```python
from build123d import *

# Parameters (mm, degrees)
F0_R     = 3
F1_DEPTH = 10
F2_R     = 2.44
F3_DEPTH = 6
F4_R     = 2.7
F5_DEPTH = 5


with BuildPart() as f1:
    # F0 (on Top) → F1 (new body)
    with BuildSketch(Plane.XY):
        with Locations((-39.492015, 19.486886)):
            Circle(F0_R)
    extrude(amount=F1_DEPTH)

    # F2 (on face) → F3 (join)
    with BuildSketch(Plane.XY.offset(10)):
        with Locations((-39.492015, 19.486886)):
            Circle(F2_R)
    extrude(amount=F3_DEPTH)

    # F4 (on face) → F5 (cut)
    with BuildSketch(Plane(origin=(0, 0, 0), x_dir=(1, 0, 0), z_dir=(0, 0, -1))):
        with Locations((-39.492015, -19.486886)):
            Circle(F4_R)
    extrude(amount=-F5_DEPTH, mode=Mode.SUBTRACT)


solid = f1.part
```
Input: part model. Units: mm. Frame: model coordinates. Give positions to 0.01 mm unless a question says otherwise; leave off trailing zeros. Order: outer loops, then holes, each group sorted by start corner. A loop starts at its lowest first (then second) coordinate and runs counter-clockwise, first axis right, second up. Notation, with made-up numbers: M -23.5,8 L 33.5,8 A16 ccw 33.5,23 Z; hole C 49,-21.5 d10. An arc over 180 degrees is marked long. One line per question, with ' | ' between items. Start each with the question number.
1. Section query B-B (y = 21.6). Return the cut outline in (x, z).
2. Section query C-C (z = 4). Return the cut outline in (x, y).
3. Section query D-D (z = 13). Return the cut outline in (x, y), and give its area (3 significant figures).
4. First-contact query: pin 1 Ø3 at (x, z) = (-41, 13) entering from -Y; pin 2 Ø1 at (x, z) = (-40, 1.5) entering from -Y. Flat tips, straight axial feed; report the tip coordinate or a pass-through.
5. Section query A-A (x = -39.05). Return the cut outline in (y, z).
6. Material intervals for probe 1 along X at (y, z) = (19.6, 1.5); probe 2 along Z at (x, y) = (-40.8, 21.75); probe 3 along X at (y, z) = (18.15, 4), sorted ascending. Write a range as [from, to].
7. Pull-direction query (X, two-part tool) for faces 1 (the face through (-37.24, 18.55, 12.96)), 2 (the face through (-40, 19, 5)), 3 (the face through (-41.635, 21.13, 2.465)), 4 (the face through (-40, 20, 16)); classes: released by +X, released by -X, zero draft, split by the parting line, or undercut.
Here are the results:
1) outline: M -41.62,0 L -41.17,0 L -41.17,5 L -37.81,5 L -37.81,0 L -37.36,0 L -37.36,10 L -38.27,10 L -38.27,16 L -40.71,16 L -40.71,10 L -41.62,10 Z
2) outline: C -39.49,19.49 d6; hole C -39.49,19.49 d5.4
3) outline: C -39.49,19.49 d4.88 | area: 18.7 mm²
4) pin 1: y = 17.05 | pin 2: y = 16.49
5) outline: M 16.52,0 L 16.82,0 L 16.82,5 L 22.15,5 L 22.15,0 L 22.45,0 L 22.45,10 L 21.89,10 L 21.89,16 L 17.09,16 L 17.09,10 L 16.52,10 Z
6) probe 1: [-42.49, -42.19], [-36.79, -36.49] | probe 2: [5, 10] | probe 3: [-42.18, -41.84], [-37.15, -36.81]
7) face 1: split by the parting line | face 2: undercut | face 3: undercut | face 4: zero draft
